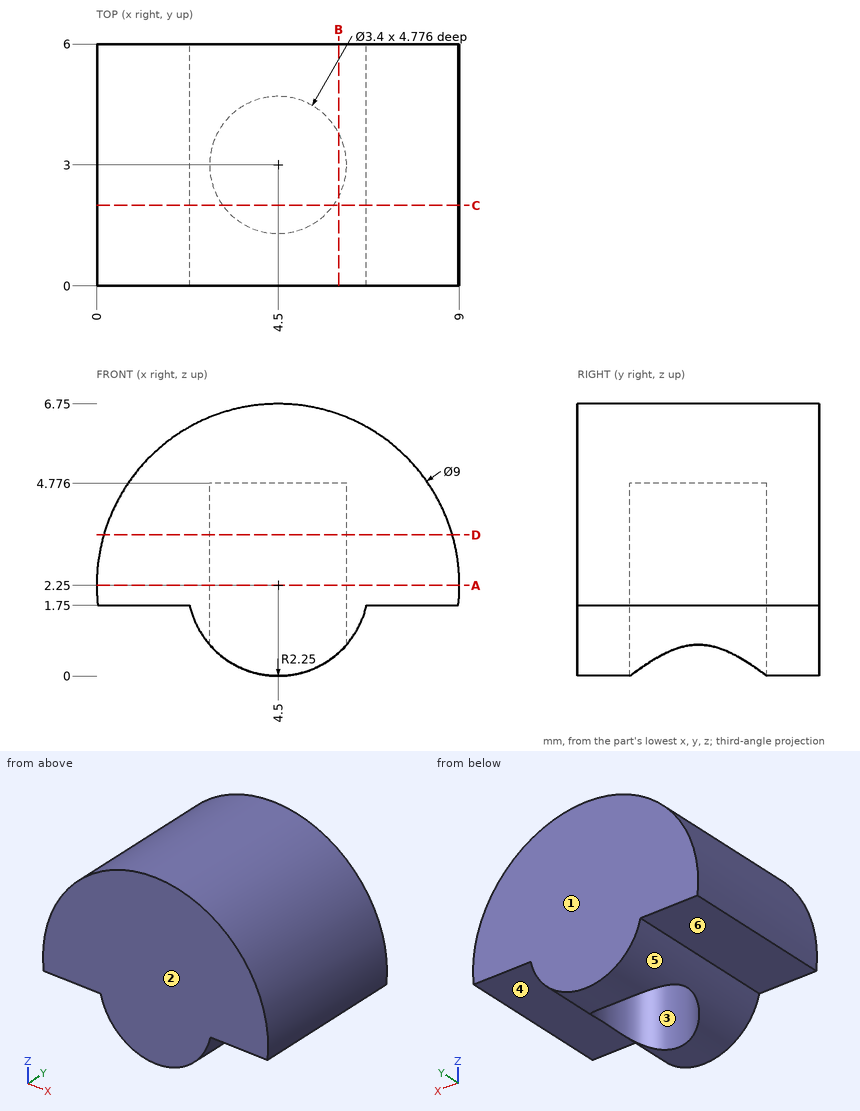
Drawing for the job (mm, zero at the part's lowest x, y, z). A direction names the side the tool comes from. Give positions to 0.01 mm unless a question says otherwise; leave off trailing zeros. Order: outer loops, then holes, each group sorted by start corner. A loop starts at its lowest first (then second) coordinate and runs counter-clockwise, first axis right, second up. Notation, with made-up numbers: (38.25, 74.5) -> (52.25, 74.5) arc R9 ccw to (52.25, 87.5) -> close; hole circle Ø10 at (59, 30). An arc over 180 degrees is marked (long way). Use one line per item in the form item = value.
(1) Saw through at C-C (y = 2). Write the cut outline in (x, z).
Solution:
outline = (0.03, 1.75) -> (2.31, 1.75) arc R2.25 ccw to (3.13, 0.47) -> (3.13, 4.78) -> (5.87, 4.78) -> (5.87, 0.47) arc R2.25 ccw to (6.69, 1.75) -> (8.97, 1.75) arc R4.5 ccw (long way) to start
(2) Saw through at B-B (x = 6). Write the cut outline in (y, z).
Solution:
outline = (0, 0.57) -> (2.2, 0.57) -> (2.2, 4.78) -> (3.8, 4.78) -> (3.8, 0.57) -> (6, 0.57) -> (6, 6.49) -> (0, 6.49) -> close
(3) Saw through at D-D (z = 3.5). Write the cut outline in (x, y), then the cut area to 3 significant figures.
Solution:
outline = (0.18, 0) -> (8.82, 0) -> (8.82, 6) -> (0.18, 6) -> close; hole circle Ø3.4 at (4.5, 3)
area = 42.8 mm²
(4) Drill centre lines: line 1 (Y direction, x = 4.5, z = 1.55); line 2 (Y direction, x = 5.75, z = 1.25); line 3 (X direction, y = 1, z = 5.5). Where is each one in solid material? Low to high. Write a range as from..to.
Solution:
line_1 = 0..1.3, 4.7..6
line_2 = 0..1.85, 4.15..6
line_3 = 1.39..7.61
(5) Saw through at A-A (z = 2.25). Write the cut outline in (x, y), then the cut area to 3 significant figures.
Solution:
outline = (0, 0) -> (9, 0) -> (9, 6) -> (0, 6) -> close; hole circle Ø3.4 at (4.5, 3)
area = 44.9 mm²
(6) Tool access for the marked faces 4, 5 and 6: list every direction of +Z, -Z, +X, -X, +Y, -Y with a clear straight run to the whole face (end or side of a thin tool).
Solution:
face_4 = -Z, +X, +Y, -Y
face_5 = -Z, +Y, -Y
face_6 = -Z, -X, +Y, -Y
(7) Pull direction Y, two halves, no side cores. Call the marked faces 1, 2 and 3: +Y half, -Y half, draft (parallel to the pull), parting line (faces both ways), or undercut.
Solution:
face_1 = +Y half
face_2 = -Y half
face_3 = undercut
(8) Flat gauge pins, fed straight in: P1, Ø2.5, axis at x = 5, y = 3.5, coming from the -Z side; P2, Ø1.1, axis at x = 8, y = 2.5, coming from the -Z side; P3, Ø1, axis at y = 2.5, z = 3.5, coming from the +X side; P4, Ø1.5, axis at x = 1, z = 5.5, coming from the -Y side. Where does each tip first touch, or does it go through?
Solution:
P1 = 0
P2 = 1.75
P3 = 8.94
P4 = 0
